Read the model definition and answer for the solid it produces. Units are mm, in the model's axes. A direction names the side the tool comes from. Round coordinates to 2 decimals unless told otherwise and drop trailing zeros.
Autodesk Inventor part; units mm, degrees
ref_plane "YZ Plane" through (0, 0, 0) normal (1, 0, 0) x (0, 1, 0)
ref_plane "XZ Plane" through (0, 0, 0) normal (0, 1, 0) x (-1, 0, 0)
ref_plane "XY Plane" through (0, 0, 0) normal (0, 0, 1) x (1, 0, 0)
sketch "Sketch2" plane through (0, 0, 0) normal (0, 1, 0) x (-1, 0, 0)
  line L0 (0, 0) -> (-81.28, 0)
  line L1 (-81.28, 0) -> (-81.28, -25.4)
  line L2 (-81.28, -25.4) -> (0, -25.4)
  line L3 (0, -25.4) -> (0, 0)
  dimension "d2" = 81.28
  dimension "d3" = 25.4
extrude "Extrusion1" add sketch "Sketch2" along normal blind 76.2
sketch "Sketch3" plane through (81.28, 0, -25.4) normal (0, 0, -1) x (-1, 0, 0)
  line L0 (81.28, 76.2) -> (0, 76.2)
  line L1 (40.64, 76.2) -> (40.64, 0)
  line L2 (0, 0) -> (0, 76.2)
  line L3 (0, 38.1) -> (81.28, 38.1)
  line L4 (81.28, 0) -> (81.28, 76.2)
  circle A0 centre (40.64, 38.1) radius 22.86
  dimension "d6" = 45.72
extrude "Extrusion2" cut sketch "Sketch3" against normal blind 25.4 contours A0 L3 L1 | L1 L3 A0 | A0 L1 L3 | L1 A0 L3
chamfer "Chamfer1" distance 20.32 distance2 76.2 1 edges at (81.28, 76.2, -12.7) measured on face at (54.1867, 76.2, -8.4667)
chamfer "Chamfer2" distance 20.32 distance2 76.2 1 edges at (0, 76.2, -12.7) measured on face at (40.6403, 76.2, -16.9333)
fillet "Fillet1" radius 27.94 2 edges at (60.9605, 76.2, -12.7) (20.3195, 76.2, -12.7)
fillet "Fillet2" radius 2.54 8 edges at (63.5, 38.1, 0) (63.5, 38.1, -25.4) (74.4578, 25.5841, 0) (6.8222, 25.5841, 0) (40.64, 71.9079, 0) (6.8222, 25.5841, -25.4) (74.4578, 25.5841, -25.4) (40.64, 71.9079, -25.4)
sketch "Sketch5" plane through (0, 0, 0) normal (0, -1, 0) x (1, 0, 0)
  line L0 (2.6288, 0) -> (78.6512, 0)
  line L1 (40.64, 0) -> (40.64, -25.4)
  line L2 (78.6512, -25.4) -> (2.6288, -25.4)
  line L3 (0, -12.7) -> (81.4991, -12.7)
  line L4 (40.7495, -12.7) -> (51.1635, -12.7)
  line L5 (51.1635, -12.7) -> (51.1635, -6.604)
  line L6 (51.1635, -6.604) -> (30.3355, -6.604)
  line L7 (30.3355, -6.604) -> (30.3355, -18.796)
  line L8 (30.3355, -18.796) -> (51.1635, -18.796)
  line L9 (51.1635, -18.796) -> (51.1635, -12.7)
  point P0 (0, 0)
  dimension "d23" = 10.414
  dimension "d24" = 6.096
  dimension "d25" = 20.828
  dimension "d26" = 12.192
extrude "Extrusion4" cut sketch "Sketch5" against normal blind 5.08
properties part number "CapStone Handle"
Q1. Straight lines are drawn through the part: probe 1 along Y at (x, z) = (40.64, -17.25); probe 2 along Z at (x, y) = (44, 4); probe 3 along X at (y, z) = (38.1, -10.5). For each, find the intervals that lie inside material, in ascending order.
Outcome:
probe 1: y = 5.08 to 15.24, 60.96 to 71.91
probe 2: z = -25.4 to -18.8, -6.6 to 0
probe 3: x = 10.16 to 17.78, 63.5 to 71.12
Q2. For faces 1 (the face through (40, 11, 0)), 2 (the face through (41, 3, -6.604)), determine the directions among +Z, -Z, +X, -X, +Y, -Y from which every point of the face is accessible in a straight line to the end or side of a thin tool.
Outcome:
face 1: +Z, +X, -X, +Y, -Y
face 2: -Y
Q3. For a pull along Z with two mould halves and no side action, classify faces 3 (the face through (73.66, 25.76, -24.64)), 4 (the face through (41, 3, -18.796)), 5 (the face through (74.553, 25.226, -12.558)), 6 (the face through (73.9, 25, -0.8)) as released by +Z, released by -Z, zero draft, split by the parting line, or undercut.
Outcome:
face 3: released by -Z
face 4: undercut
face 5: zero draft
face 6: released by +Z
Q4. Flat-ended cylindrical pins translate along their axes: pin 1 (5.5 mm diameter, centred on y = 3, z = -11, fed in from -X); pin 2 (2.5 mm diameter, centred on y = 2.5, z = -13.5, fed in from +X); pin 3 (4 mm diameter, centred on y = 53, z = -2.5, fed in from +X). Find the tip coordinate at first contact, or state that the pin passes through.
Outcome:
pin 1: stops at x = 0.07
pin 2: stops at x = 80.95
pin 3: stops at x = 67.68
